Can you work these out from the drawing? Everything is in mm from the part's minimum corner. Give positions to 0.01 mm unless a question says otherwise; leave off trailing zeros. Write each loop counter-clockwise with the first axis right and the second up, starting at its lowest first coordinate (ties: lowest second). Pieces come first, ordered by that corner, then holes. Notation, with made-up numbers: (-12, -32) - (46, -32) arc R22 ccw to (46, -15) - close; hole circle Ø2 at (56.25, 4). An arc over 180 degrees is marked (long way). Answer in a Markdown table with one row per item.
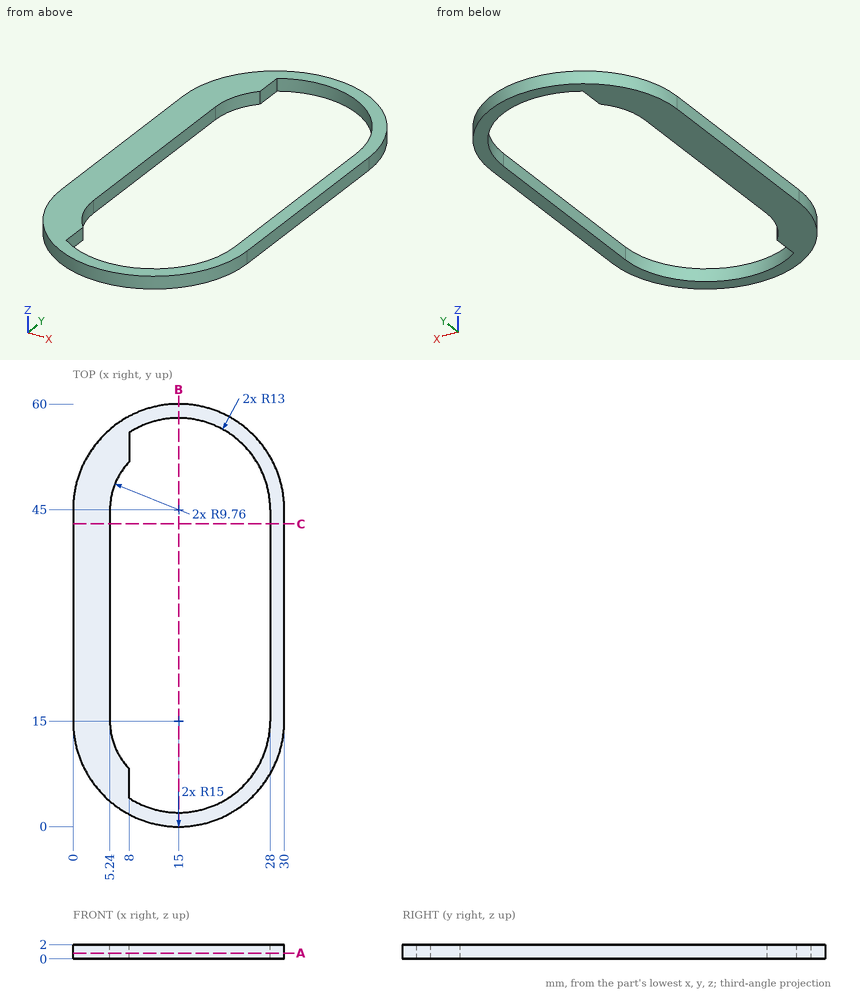
1) Imagine slicing it at B-B (x = 15). List the corners of the cut face in (y, z) for me, then the cut area to 3 significant figures.
Check values:
| item | result |
|---|---|
| outline | (0, 0) - (2, 0) - (2, 2) - (0, 2) - close; (58, 0) - (60, 0) - (60, 2) - (58, 2) - close |
| area | 8.00 mm2 |
2) If I drill on line 1 (X direction, y = 19, z = 1.55); line 2 (Y direction, x = 15, z = 0.4); line 3 (X direction, y = 46, z = 1.9), over which ranges is the centre line in solid material (lowest first)?
Check values:
| item | result |
|---|---|
| line 1 | x = 0 to 5.24, 28 to 30 |
| line 2 | y = 0 to 2, 58 to 60 |
| line 3 | x = 0.03 to 5.29, 27.96 to 29.97 |
3) Will these pins go through, and if not, where does the flat tip stop? P1, Ø8, axis at x = 3.5, y = 45, coming from the -Z side; P2, Ø0.6, axis at y = 7, z = 1, coming from the +X side.
Check values:
| item | result |
|---|---|
| P1 | stops at z = 0 |
| P2 | stops at x = 27.87 |
4) Imagine slicing it at A-A (z = 0.8). List the corners of the cut face in (x, y) for me, then the cut area to 3 significant figures.
Check values:
| item | result |
|---|---|
| outline | (0, 15) arc R15 ccw to (30, 15) - (30, 45) arc R15 ccw to (0, 45) - close; hole (5.24, 15) arc R9.76 ccw to (8, 8.2) - (8, 4.05) arc R13 ccw to (28, 15) - (28, 45) arc R13 ccw to (8, 55.95) - (8, 51.8) arc R9.76 ccw to (5.24, 45) - close |
| area | 460 mm2 |
5) Imagine slicing it at C-C (y = 43). List the corners of the cut face in (x, z) for me, then the cut area to 3 significant figures.
Check values:
| item | result |
|---|---|
| outline | (0, 0) - (5.24, 0) - (5.24, 2) - (0, 2) - close; (28, 0) - (30, 0) - (30, 2) - (28, 2) - close |
| area | 14.5 mm2 |
